```python
from build123d import *

# Parameters (mm, degrees)
CHAMFER1_SIZE       = 0.3
SKETCH2_W           = 0.855522376
SKETCH2_H           = 3.315149208
BOSS_EXTRUDE1_DEPTH = 5
SKETCH3_R           = 0.78364852
CUT_EXTRUDE1_DEPTH  = 12
FILLET1_R           = 1


with BuildPart() as part:
    # Sketch1 → Revolve1 (revolve)
    with BuildSketch(Plane.XY, mode=Mode.PRIVATE) as revolve1_sk:
        with BuildLine():
            Line((0, 0), (2.5, 0))
            ThreePointArc((2.5, 0), (4.614619792, -0.739532292), (6, -2.5))
            Line((6, -2.5), (6, -3))
            Line((6, -3), (7.5, -3))
            Line((7.5, -3), (9, -5.5))
            Line((9, -5.5), (9, -8.5))
            Line((9, -8.5), (6, -8.5))
            Line((6, -8.5), (6, -18))
            Line((6, -18), (0, -18))
            Line((0, -18), (0, 0))
        make_face()
    revolve(revolve1_sk.sketch.rotate(Axis((0, 0, 0), (0, -1, 0)), 90), axis=Axis((0, 0, 0), (0, -1, 0)))

    # Chamfer1
    chamfer1_edges = [part.edges().sort_by_distance(p)[0] for p in [
        (0, -8.5, -6),
        (0, -18, -6),
        (0, -8.5, -9),
    ]]
    chamfer(chamfer1_edges, length=CHAMFER1_SIZE)

    # Sketch2 → Boss-Extrude1 (add)
    with BuildSketch(Plane.XZ.offset(18)):
        with Locations((2.709154191, 0)):
            Rectangle(SKETCH2_W, SKETCH2_H)
        with Locations((-2.709154191, 0)):
            Rectangle(SKETCH2_W, SKETCH2_H)
    extrude(amount=BOSS_EXTRUDE1_DEPTH)

    # Sketch3 → Cut-Extrude1 (cut)
    with BuildSketch(Plane.ZY.offset(3.136915379)):
        with Locations((0, -21.270184358)):
            Circle(SKETCH3_R)
    extrude(amount=-CUT_EXTRUDE1_DEPTH, mode=Mode.SUBTRACT)

    # Fillet1
    fillet1_edges = [part.edges().sort_by_distance(p)[0] for p in [
        (2.709154191, -23, 1.657574604),
        (2.709154191, -23, -1.657574604),
        (-2.709154191, -23, 1.657574604),
        (-2.709154191, -23, -1.657574604),
    ]]
    fillet(fillet1_edges, radius=FILLET1_R)


solid = part.part
```
Geometry check sheet. Reference: the model listing, model coordinates, mm. A direction names the side the tool comes from. Round coordinates to 2 decimals unless told otherwise and drop trailing zeros. Loops run counter-clockwise (first coordinate to the right, second up) from the corner with the lowest first, then second, coordinate; pieces in that order, holes last. Notation, with made-up numbers: (26, 56) - (64, 56) arc R19 cw to (64, 70) - close; hole circle Ø10 at (36, 39.5). An arc over 180 degrees is marked (long way). Use a Markdown table: item, result.
Q1. Cross-section at B-B on y = -12.5. Record the cut outline in (x, z), plus the area to 3 significant figures.
Solutions:
| item | result |
|---|---|
| outline | circle Ø12 at (0, 0) |
| area | 113 mm2 |
Q2. Go/stop test with flat-tipped pins: P1, Ø1, axis at y = -19.5, z = -0.5, coming from the +X side; P2, Ø5, axis at x = -7, y = -4.5, coming from the -Z side; P3, Ø0.9, axis at x = 3, y = -20, coming from the +Z side; P4, Ø1.5, axis at y = -13.5, z = -7, coming from the +X side. Record where each tip stops, or that it passes through.
Solutions:
| item | result |
|---|---|
| P1 | stops at x = 3.14 |
| P2 | stops at z = -7.67 |
| P3 | stops at z = 1.66 |
| P4 | passes through |
Q3. Draft check along X on faces 1 (the cylindrical face through (-6.083, -6.869, -6.633)), 2 (the flat face through (-2.281, -20, 0)), 3 (the cylindrical face through (-2.72, -20.61, 0.42)). Enter one of: released by +X, released by -X, zero draft, split by the parting line, or undercut.
Solutions:
| item | result |
|---|---|
| face 1 | split by the parting line |
| face 2 | undercut |
| face 3 | zero draft |
Q4. Access from +Z, -Z, +X, -X, +Y, -Y to the whole of each face (thin tool, end or side, straight path). Record for faces 4 (the flat face through (-3, -8.5, 6)), 5 (the flat face through (2.7, -20, -1.658)), 6 (the flat face through (2.281, -20, 0)).
Solutions:
| item | result |
|---|---|
| face 4 | -Y |
| face 5 | -Z, +X, -X, -Y |
| face 6 | +Z, -Z, -Y |
Q5. Cross-section at A-A on z = 0. State how many separate pieces and enclosed holes the cut face has, plus the area to 3 significant figures.
Solutions:
| item | result |
|---|---|
| separate pieces | 3 |
| enclosed holes | 0 |
| area | 246 mm2 |
Q6. Material ranges on line 1 (X direction, y = -20, z = 1); line 2 (Y direction, x = 2.95, z = 0); line 3 (Y direction, x = 5, z = 4.25), recorded low to high.
Solutions:
| item | result |
|---|---|
| line 1 | x = -3.14 to -2.28, 2.28 to 3.14 |
| line 2 | y = -23 to -22.05, -20.49 to -0.05 |
| line 3 | y = -8.5 to -3 |
